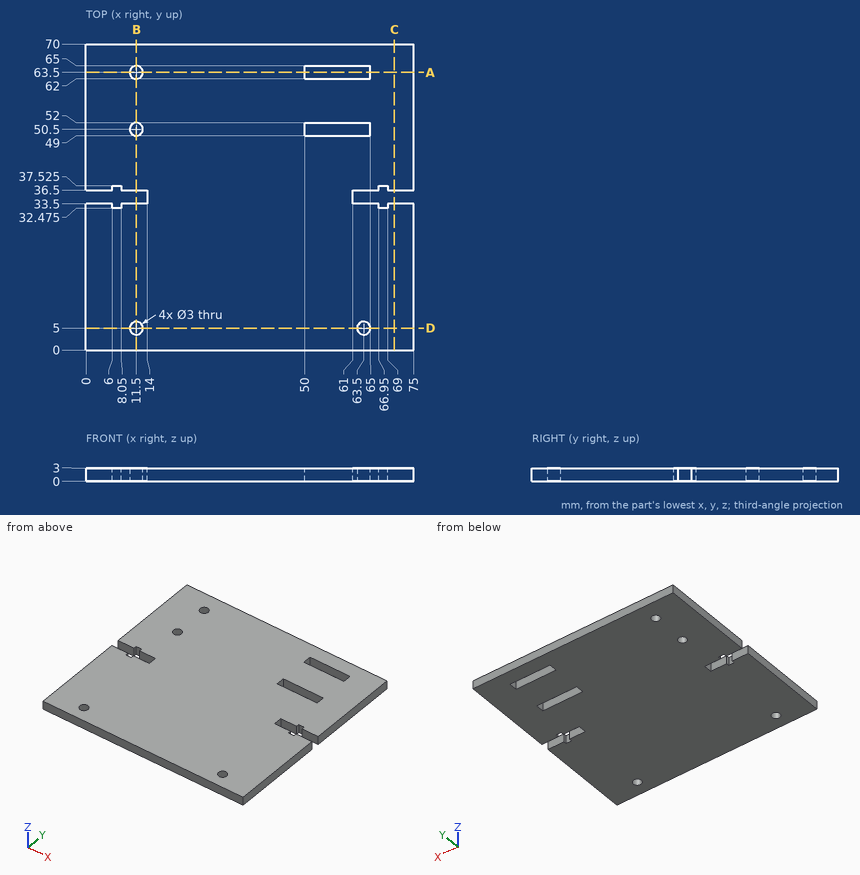
Check sheet for the drawn part. Datum: minimum x, y, z corner. Units: mm. Coordinates: 2 decimals unless noted, no trailing zeros. Order: outer loops, then holes, each group sorted by start corner. A loop starts at its lowest first (then second) coordinate and runs counter-clockwise, first axis right, second up. Notation, with made-up numbers: (88, 71.5) -> (111, 71.5) arc R13 ccw to (111, 78.5) -> close; hole circle Ø4 at (76.25, 22). An arc over 180 degrees is marked (long way). Write each question's results on one line, items separated by ' | '. Start each with the question number.
1) Material ranges on line 1 along Y through (x, z) = (11.5, 2.15); line 2 along Y through (x, z) = (4, 2.8); line 3 along X through (y, z) = (63, 1.3), recorded low to high.
2) Section check B-B (x = 11.5). Enter the section's corners in (y, z).
3) Section check D-D (y = 5). Enter the section's corners in (x, z), and give its area (3 significant figures).
4) Section check C-C (x = 70.5). Enter the section's corners in (y, z).
5) Section check A-A (y = 63.5). Enter the section's corners in (x, z).
Checked values:
1) line 1: 0 to 3.5, 6.5 to 33.5, 36.5 to 49, 52 to 62, 65 to 70 | line 2: 0 to 33.5, 36.5 to 70 | line 3: 0 to 10.09, 12.91 to 50, 65 to 75
2) outline: (0, 0) -> (3.5, 0) -> (3.5, 3) -> (0, 3) -> close; (6.5, 0) -> (33.5, 0) -> (33.5, 3) -> (6.5, 3) -> close; (36.5, 0) -> (49, 0) -> (49, 3) -> (36.5, 3) -> close; (52, 0) -> (62, 0) -> (62, 3) -> (52, 3) -> close; (65, 0) -> (70, 0) -> (70, 3) -> (65, 3) -> close
3) outline: (0, 0) -> (10, 0) -> (10, 3) -> (0, 3) -> close; (13, 0) -> (62, 0) -> (62, 3) -> (13, 3) -> close; (65, 0) -> (75, 0) -> (75, 3) -> (65, 3) -> close | area: 207 mm²
4) outline: (0, 0) -> (33.5, 0) -> (33.5, 3) -> (0, 3) -> close; (36.5, 0) -> (70, 0) -> (70, 3) -> (36.5, 3) -> close
5) outline: (0, 0) -> (10, 0) -> (10, 3) -> (0, 3) -> close; (13, 0) -> (50, 0) -> (50, 3) -> (13, 3) -> close; (65, 0) -> (75, 0) -> (75, 3) -> (65, 3) -> close
